from build123d import *

# Parameters (mm, degrees)
F1_DEPTH = 12
F2_SIZE2 = 3.4641016151
F2_SIZE  = 2
F3_T     = -2.9


with BuildPart() as f1:
    # F0 (on Top) → F1 (new body)
    with BuildSketch(Plane.XY):
        with BuildLine():
            ThreePointArc((-66, -51), (-61.6066017178, -61.6066017178), (-51, -66))
            Line((-51, -66), (51, -66))
            ThreePointArc((51, -66), (61.6066017178, -61.6066017178), (66, -51))
            Line((66, -51), (66, 51))
            ThreePointArc((66, 51), (61.6066017178, 61.6066017178), (51, 66))
            Line((51, 66), (-51, 66))
            ThreePointArc((-51, 66), (-61.6066017178, 61.6066017178), (-66, 51))
            Line((-66, 51), (-66, -51))
        make_face()
    extrude(amount=F1_DEPTH)

    # F2
    f2_edges = [f1.edges().sort_by_distance(p)[0] for p in [
        (0, -66, 12),
    ]]
    f2_side = f1.faces().sort_by_distance((0, 0, 12))[0]
    chamfer(f2_edges, length=F2_SIZE, length2=F2_SIZE2, reference=f2_side)

    # F3
    f3_openings = [f1.faces().sort_by_distance(p)[0] for p in [
        (0, 0, 0),
    ]]
    offset(amount=F3_T, openings=f3_openings)


solid = f1.part
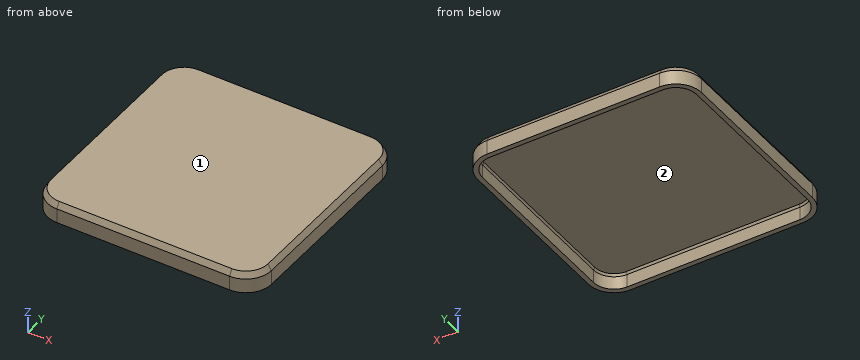
The listing builds one solid part. Answer for the finished solid, in the listing's coordinates (mm). Face numbers are marked on the shaded views. Give positions to 0.01 mm unless a question says otherwise; leave off trailing zeros. Order: outer loops, then holes, each group sorted by start corner. A loop starts at its lowest first (then second) coordinate and runs counter-clockwise, first axis right, second up. Notation, with made-up numbers: (2.25, 76.25) - (29.25, 76.25) arc R20 ccw to (29.25, 91.25) - close; hole circle Ø8 at (83, 57.25). An arc over 180 degrees is marked (long way). Use one line per item in the form item = value.
1) Find section C-C on z = 5.75. Determine the outline of the cut face in (x, y).
Verdict:
outline = (-66, -51) arc R15 ccw to (-51, -66) - (51, -66) arc R15 ccw to (66, -51) - (66, 51) arc R15 ccw to (51, 66) - (-51, 66) arc R15 ccw to (-66, 51) - close; hole (-63.1, -51) arc R12.1 ccw to (-51, -63.1) - (51, -63.1) arc R12.1 ccw to (63.1, -51) - (63.1, 51) arc R12.1 ccw to (51, 63.1) - (-51, 63.1) arc R12.1 ccw to (-63.1, 51) - close
2) Consider probe 1 along Y at (x, z) = (-12, 2.25); probe 2 along Z at (x, y) = (42.5, -37). Determine where each line is inside the solid, lowest interval first. Write a range as [from, to].
Verdict:
probe_1 = [-66, -63.1], [63.1, 66]
probe_2 = [9.1, 12]
3) The mould has two halves that part along Y. Classify the marked faces 1 and 2: released by +Y, released by -Y, zero draft, split by the parting line, or undercut.
Verdict:
face_1 = zero draft
face_2 = undercut
4) Find section A-A on x = -46.5. Determine the outline of the cut face in (y, z), and give its area (3 significant figures).
Verdict:
outline = (-66, 0) - (-63.1, 0) - (-63.1, 7.76) - (-62.33, 9.1) - (62.33, 9.1) - (63.1, 7.76) - (63.1, 0) - (66, 0) - (66, 8.54) - (64, 12) - (-64, 12) - (-66, 8.54) - close
area = 430 mm^2
5) This flat-tipped pin is pushed along its axis until it touches: pin 1 (3 mm diameter, centred on x = -23, y = 15.5, fed in from -Z). Where does it stop, or does it pass through?
Verdict:
pin_1 = 9.1
